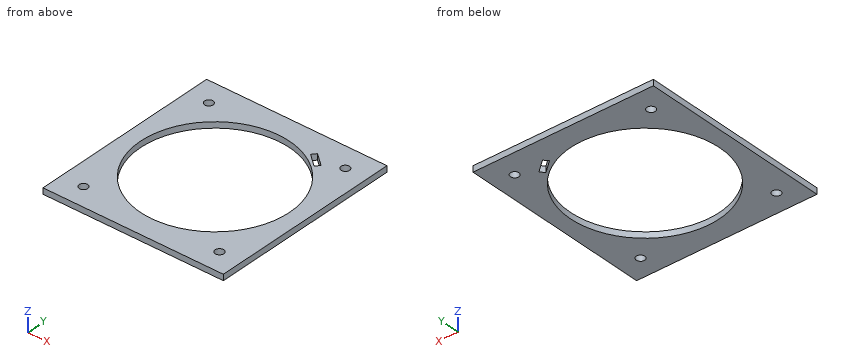
from build123d import *

# Parameters (mm, degrees)
SKETCH1_W               = 84.8
SKETCH1_H               = 90.5
BOSS_EXTRUDE1_DEPTH     = 2.794
CUT_EXTRUDE1_DEPTH      = 125.05279697
CUT_EXTRUDE1_DEPTH_BACK = 125.05279697
SKETCH2_R               = 2
CUT_EXTRUDE2_DEPTH      = 125.05279697
CUT_EXTRUDE2_DEPTH_BACK = 125.05279697
SKETCH3_R               = 1.7145
SKETCH4_R               = 35
CUT_EXTRUDE3_DEPTH      = 10
CUT_EXTRUDE4_DEPTH      = 10


with BuildPart() as part:
    # Sketch1 → Boss-Extrude1 (new body)
    with BuildSketch(Plane.XY):
        with Locations((42.4, -45.25)):
            Rectangle(SKETCH1_W, SKETCH1_H)
    extrude(amount=BOSS_EXTRUDE1_DEPTH)

    # Sketch2 → Cut-Extrude1 (cut, two sides: drawn at the far end of the back side and taken through both)
    with BuildSketch(Plane.XY.offset(2.794).offset(-CUT_EXTRUDE1_DEPTH_BACK)):
        with Locations((10.31500695, -10.904966862)):
            Circle(SKETCH2_R)
        with Locations((74.48499305, -10.904966862)):
            Circle(SKETCH2_R)
        with Locations((74.48499305, -80.5)):
            Circle(SKETCH2_R)
        with Locations((10.53300695, -80.5)):
            Circle(SKETCH2_R)
    extrude(amount=CUT_EXTRUDE1_DEPTH + CUT_EXTRUDE1_DEPTH_BACK, mode=Mode.SUBTRACT)

    # Sketch3 → Cut-Extrude2 (cut, two sides: drawn at the far end of the back side and taken through both)
    with BuildSketch(Plane(origin=(0, 0, 0), x_dir=(-1, 0, 0), z_dir=(0, 0, -1)).offset(-CUT_EXTRUDE2_DEPTH_BACK)):
        with Locations((-42.4, -45.25)):
            Circle(SKETCH3_R)
    extrude(amount=CUT_EXTRUDE2_DEPTH + CUT_EXTRUDE2_DEPTH_BACK, mode=Mode.SUBTRACT)

    # Sketch4 → Cut-Extrude3 (cut)
    with BuildSketch(Plane(origin=(0, 0, 0), x_dir=(-1, 0, 0), z_dir=(0, 0, -1))):
        with Locations((-42.4, -45.25)):
            Circle(SKETCH4_R)
    extrude(amount=-CUT_EXTRUDE3_DEPTH, mode=Mode.SUBTRACT)

    # Sketch5 → Cut-Extrude4 (cut)
    with BuildSketch(Plane.XY.offset(2.794)):
        Polygon((60.865488083, -10.264365241), (66.70274674, -15.162406827), (65.070066211, -17.108159712), (59.232807555, -12.210118127), align=None)
    extrude(amount=-CUT_EXTRUDE4_DEPTH, mode=Mode.SUBTRACT)


solid = part.part
Read the model definition and answer for the solid it produces. Units are mm, in the model's axes. Coordinates: 2 decimals unless noted, no trailing zeros. Order: outer loops, then holes, each group sorted by start corner. A loop starts at its lowest first (then second) coordinate and runs counter-clockwise, first axis right, second up. Notation, with made-up numbers: M 30.5,2 L 70.5,2 A14 cw 70.5,22 Z; hole C 37.25,89 d3. An arc over 180 degrees is marked long. Put each result on its own line as item: value. Start each with the question number.
Item 1: Consider probe 1 along X at (y, z) = (-80.5, 2.2) (3 decimals); probe 2 along Y at (x, z) = (62.5, 1.45); probe 3 along Y at (x, z) = (42.4, 2.1). Determine where each line is inside the solid, lowest interval first. Write a range as [from, to].
Item 2: Section C-C, the plane z = 1.15 is taken. Determine the outline of the cut face in (x, y) (3 decimals).
Item 3: Section A-A, the plane y = -45.25 is taken. Determine the outline of the cut face in (x, z), plus the area to 3 significant figures.
Item 4: Section D-D, the plane x = 73.5 is taken. Determine the outline of the cut face in (y, z).
Item 5: Section B-B, the plane x = 42.4 is taken. Determine the outline of the cut face in (y, z), plus the area to 3 significant figures.
Computed:
1. probe 1: x = [0, 8.533], [12.533, 72.485], [76.485, 84.8]
1. probe 2: y = [-90.5, -73.9], [-16.6, -14.95], [-11.64, 0]
1. probe 3: y = [-90.5, -80.25], [-10.25, 0]
2. outline: M 0,-90.5 L 84.8,-90.5 L 84.8,0 L 0,0 Z; hole C 42.4,-45.25 d70; hole C 10.315,-10.905 d4; hole C 10.533,-80.5 d4; hole M 59.233,-12.21 L 65.07,-17.108 L 66.703,-15.162 L 60.865,-10.264 Z; hole C 74.485,-80.5 d4; hole C 74.485,-10.905 d4
3. outline: M 0,0 L 7.4,0 L 7.4,2.79 L 0,2.79 Z; M 77.4,0 L 84.8,0 L 84.8,2.79 L 77.4,2.79 Z
3. area: 41.4 mm2
4. outline: M -90.5,0 L -82.24,0 L -82.24,2.79 L -90.5,2.79 Z; M -78.76,0 L -61.31,0 L -61.31,2.79 L -78.76,2.79 Z; M -29.19,0 L -12.65,0 L -12.65,2.79 L -29.19,2.79 Z; M -9.16,0 L 0,0 L 0,2.79 L -9.16,2.79 Z
5. outline: M -90.5,0 L -80.25,0 L -80.25,2.79 L -90.5,2.79 Z; M -10.25,0 L 0,0 L 0,2.79 L -10.25,2.79 Z
5. area: 57.3 mm2
